The model under review builds one solid part; all positions refer to its coordinate system, in mm. A direction names the side the tool comes from. Round coordinates to 2 decimals unless told otherwise and drop trailing zeros. Write each loop counter-clockwise with the first axis right and the second up, starting at its lowest first coordinate (ties: lowest second). Pieces come first, ordered by that corner, then holes. Notation, with made-up numbers: (17.25, -27) -> (62.25, -27) arc R27 ccw to (62.25, -4) -> close; hole circle Ø4 at (81.5, 64). An arc over 180 degrees is marked (long way). Return JSON: item names as keys, results as strings. Group by question number.
1. Tool access review of faces 1 (the flat face through (11, -3, -15)), 2 (the flat face through (71, -2, 12)): name each direction out of +Z, -Z, +X, -X, +Y, -Y from which nothing blocks a thin tool from reaching the whole face with its end or side.
2. Clearance check with flat-ended pins moving along their axes: P1, Ø3, axis at y = 7.5, z = 6.5, coming from the +X side; P2, Ø6, axis at x = 43, z = 10, coming from the +Y side; P3, Ø16, axis at x = 72, z = 0, coming from the +Y side. State where each tip first meets the part, or that it passes through.
3. Mouldability with a two-part tool opening along Y and no side actions: class faces 3 (the flat face through (11, -3, 15)), 4 (the flat face through (4, -16, 0)), 5 (the cylindrical face through (3, -7, -1)), 6 (the cylindrical face through (12.35, 0.33, -0.21)) as pulls with the +Y half, pulls with the -Y half, needs draft (parallel to the pull), parting line crosses it, or undercut.
4. Take a section at B-B, the plane y = 5. Give the number of separate pieces and of enclosed holes in the cut face, then the cut area to 3 significant figures.
5. Take a section at A-A, the plane x = 71. Write out the cut boundary in (y, z), then the cut area to 3 significant figures.
6. Take a section at C-C, the plane x = -50. Write out the cut boundary in (y, z).
7. For line 1 along Z through (x, y) = (17, -7); line 2 along Z through (x, y) = (75, 6.5); line 3 along X through (y, z) = (-0.5, -11.5), list the stretches that pass through material, from the lowest coordinate up. Write a range as from..to.
from build123d import *

# Parameters (mm, degrees)
CYLINDER006_R               = 2.5
CYLINDER006_DEPTH           = 35
BOX004_W                    = 20
BOX004_H                    = 52
BOX004_DEPTH                = 24
CYLINDER005_R               = 5
CYLINDER005_DEPTH           = 20
CYLINDER005_PLACEMENT_ANGLE = 46
CHAMFER001_SIZE             = 4
CYLINDER004_R               = 2.5
CYLINDER004_DEPTH           = 100
CYLINDER004_PLACEMENT_ANGLE = 46
CYLINDER002_R               = 2
CYLINDER002_DEPTH           = 100
BOX_W                       = 10
BOX_H                       = 40
BOX_DEPTH                   = 100
CYLINDER001_R               = 13
CYLINDER001_DEPTH           = 56
CYLINDER_R                  = 230
CYLINDER_DEPTH              = 100
FUSION_PLACEMENT_ANGLE      = 52.3
FUSION001_PLACEMENT_ANGLE   = 22.4
BOX001_W                    = 49
BOX001_H                    = 54
BOX001_DEPTH                = 100
CYLINDER003_R               = 5
CYLINDER003_DEPTH           = 300
TORUS_R                     = 5
BOX003_W                    = 39
BOX003_H                    = 50
BOX003_DEPTH                = 42
BOX002_W                    = 209
BOX002_H                    = 50
BOX002_DEPTH                = 30
CHAMFER_SIZE                = 15
FILLET_R                    = 2
CHAMFER002_SIZE             = 0.5
CHAMFER003_SIZE             = 1
CHAMFER004_SIZE             = 0.5
CHAMFER005_SIZE             = 1
CHAMFER006_SIZE             = 0.5


with BuildPart() as cylinder006:
    # Cylinder006 → Cylinder006 (new body)
    with BuildSketch(Plane(origin=(10, 0, 3), x_dir=(1, 0, 0), z_dir=(0, -1, 0))):
        Circle(CYLINDER006_R)
    extrude(amount=CYLINDER006_DEPTH)


with BuildPart() as fusion005:
    # Box004 → Box004 (new body)
    with BuildSketch(Plane(origin=(0, -13, -12), x_dir=(1, 0, 0), z_dir=(0, 0, 1))):
        with Locations((10, 26)):
            Rectangle(BOX004_W, BOX004_H)
    extrude(amount=BOX004_DEPTH)

    # Fusion005: union Cylinder006
    add(cylinder006.part)


with BuildPart() as fusion005_1:
    # Fusion005 placement: moved
    add(fusion005.part.moved(Location((61, 0, 0))))


with BuildPart() as chamfer001:
    # Cylinder005 → Cylinder005 (new body)
    with BuildSketch(Plane.XY):
        Circle(CYLINDER005_R)
    extrude(amount=CYLINDER005_DEPTH)


with BuildPart() as chamfer001_1:
    # Cylinder005 placement: moved
    add(chamfer001.part.moved(Location((-52, -8, -20))).rotate(Axis((-52, -8, -20), (0, -1, 0)), CYLINDER005_PLACEMENT_ANGLE))

    # Chamfer001
    chamfer001_edges = [chamfer001_1.edges().sort_by_distance(p)[0] for p in [
        (-69.860088, -8, -9.703532),
    ]]
    chamfer(chamfer001_edges, length=CHAMFER001_SIZE)


with BuildPart() as chamfer001_2:
    # Chamfer001 placement: moved
    add(chamfer001_1.part.moved(Location((-14, 0, 0))))


with BuildPart() as cylinder004:
    # Cylinder004 → Cylinder004 (new body)
    with BuildSketch(Plane.XY):
        Circle(CYLINDER004_R)
    extrude(amount=CYLINDER004_DEPTH)


with BuildPart() as cylinder004_1:
    # Cylinder004 placement: moved
    add(cylinder004.part.moved(Location((-66, -8, -20))).rotate(Axis((-66, -8, -20), (0, -1, 0)), CYLINDER004_PLACEMENT_ANGLE))


with BuildPart() as cylinder002:
    # Cylinder002 → Cylinder002 (new body)
    with BuildSketch(Plane(origin=(106, 11, -34), x_dir=(1, 0, 0), z_dir=(0, 0, 1))):
        Circle(CYLINDER002_R)
    extrude(amount=CYLINDER002_DEPTH)


with BuildPart() as obj1:
    # Box → Box (new body)
    with BuildSketch(Plane(origin=(1000, -30, -50), x_dir=(1, 0, 0), z_dir=(0, 0, 1))):
        with Locations((5, 20)):
            Rectangle(BOX_W, BOX_H)
    extrude(amount=BOX_DEPTH)


with BuildPart() as cylinder001:
    # Cylinder001 → Cylinder001 (new body)
    with BuildSketch(Plane.XZ.offset(-6)):
        Circle(CYLINDER001_R)
    extrude(amount=CYLINDER001_DEPTH)


with BuildPart() as fusion001:
    # Cylinder → Cylinder (new body)
    with BuildSketch(Plane(origin=(0, 230, -50), x_dir=(1, 0, 0), z_dir=(0, 0, 1))):
        Circle(CYLINDER_R)
    extrude(amount=CYLINDER_DEPTH)

    # Fusion: union Cylinder001
    add(cylinder001.part)


with BuildPart() as fusion001_1:
    # Fusion placement: moved
    add(fusion001.part.moved(Location((181.981413, 89.348781, 0))).rotate(Axis((181.981413, 89.348781, 0), (0, 0, 1)), FUSION_PLACEMENT_ANGLE))

    # Fusion001: union obj1
    add(obj1.part)


with BuildPart() as fusion001_2:
    # Fusion001 placement: moved
    add(fusion001_1.part.moved(Location((-87.646187, 17.354412, 0))).rotate(Axis((-87.646187, 17.354412, 0), (0, 0, -1)), FUSION001_PLACEMENT_ANGLE))


with BuildPart() as fusion002:
    # Box001 → Box001 (new body)
    with BuildSketch(Plane(origin=(-141, -28, -50), x_dir=(1, 0, 0), z_dir=(0, 0, 1))):
        with Locations((24.5, 27)):
            Rectangle(BOX001_W, BOX001_H)
    extrude(amount=BOX001_DEPTH)

    # Fusion002: union Fusion001
    add(fusion001_2.part)


with BuildPart() as cylinder003:
    # Cylinder003 → Cylinder003 (new body)
    with BuildSketch(Plane(origin=(-53, -7, 0), x_dir=(0, 0, -1), z_dir=(1, 0, 0))):
        Circle(CYLINDER003_R)
    extrude(amount=CYLINDER003_DEPTH)


with BuildPart() as torus:
    # Torus → Torus (revolve)
    with BuildSketch(Plane(origin=(-53, -7, 30), x_dir=(1, 0, 0), z_dir=(0, 0, -1))):
        with Locations((30, 0)):
            Circle(TORUS_R)
    revolve(axis=Axis((-53, -7, 30), (0, -1, 0)))


with BuildPart() as holes:
    # Box003 → Box003 (new body)
    with BuildSketch(Plane(origin=(-92, -16, -15), x_dir=(1, 0, 0), z_dir=(0, 0, 1))):
        with Locations((19.5, 25)):
            Rectangle(BOX003_W, BOX003_H)
    extrude(amount=BOX003_DEPTH)

    # Common: intersect Torus
    add(torus.part, mode=Mode.INTERSECT)

    # Fusion006: union Cylinder003
    add(cylinder003.part)


with BuildPart() as holes_1:
    # Fusion006 placement: moved
    add(holes.part.moved(Location((0, 0, -6))))

    # Fusion007: union Fusion005, Chamfer001, Cylinder004, Cylinder002, Fusion002
    add(fusion005_1.part)
    add(chamfer001_2.part)
    add(cylinder004_1.part)
    add(cylinder002.part)
    add(fusion002.part)


with BuildPart() as chamfer006:
    # Box002 → Box002 (new body)
    with BuildSketch(Plane(origin=(-92, -16, -15), x_dir=(1, 0, 0), z_dir=(0, 0, 1))):
        with Locations((104.5, 25)):
            Rectangle(BOX002_W, BOX002_H)
    extrude(amount=BOX002_DEPTH)

    # Chamfer
    chamfer_edges = [chamfer006.edges().sort_by_distance(p)[0] for p in [
        (117, -16, 0),
    ]]
    chamfer(chamfer_edges, length=CHAMFER_SIZE)

    # Cut: cut holes
    add(holes_1.part, mode=Mode.SUBTRACT)

    # Fillet
    fillet_edges = [chamfer006.edges().sort_by_distance(p)[0] for p in [
        (117, 31.982324, 13.856394),
        (117, 31.982324, -13.856394),
        (-92, 19.201518, 0),
    ]]
    fillet(fillet_edges, radius=FILLET_R)

    # Chamfer002
    chamfer002_edges = [chamfer006.edges().sort_by_distance(p)[0] for p in [
        (68.5, -16, 3),
        (68.5, -13, 3),
    ]]
    chamfer(chamfer002_edges, length=CHAMFER002_SIZE)

    # Chamfer003
    chamfer003_edges = [chamfer006.edges().sort_by_distance(p)[0] for p in [
        (-86.823069, -7, 15),
        (110.998637, -7.001363, -1),
    ]]
    chamfer(chamfer003_edges, length=CHAMFER003_SIZE)

    # Chamfer004
    chamfer004_edges = [chamfer006.edges().sort_by_distance(p)[0] for p in [
        (104, 11, 15),
        (104, 11, -15),
    ]]
    chamfer(chamfer004_edges, length=CHAMFER004_SIZE)

    # Chamfer005
    chamfer005_edges = [chamfer006.edges().sort_by_distance(p)[0] for p in [
        (-78.375432, -8.003753, -15),
    ]]
    chamfer(chamfer005_edges, length=CHAMFER005_SIZE)

    # Chamfer006
    chamfer006_edges = [chamfer006.edges().sort_by_distance(p)[0] for p in [
        (-92, -7.998647, 1.6325),
    ]]
    chamfer(chamfer006_edges, length=CHAMFER006_SIZE)


solid = chamfer006.part
Output:
{
 "1": {"face 1": "-Z, +X, -X, +Y, -Y", "face 2": "+Y"},
 "2": {"P1": "stops at x = 116.38", "P2": "stops at y = 4.65", "P3": "stops at y = -13"},
 "3": {"face 3": "needs draft", "face 4": "pulls with the -Y half", "face 5": "undercut", "face 6": "pulls with the +Y half"},
 "4": {"separate pieces": "2", "enclosed holes": "1", "area": "2,900 mm^2"},
 "5": {"outline": "(-16, -15) -> (11.23, -15) -> (11.23, -12) -> (-13, -12) -> (-13, 0) -> (-13.5, 0.5) -> (-15.5, 0.5) -> (-16, 0) -> close; (-16, 6) -> (-15.5, 5.5) -> (-13.5, 5.5) -> (-13, 6) -> (-13, 12) -> (11.23, 12) -> (11.23, 15) -> (-16, 15) -> close", "area": "220 mm^2"},
 "6": {"outline": "(-16, -15) -> (5.5, -15) -> (5.5, 15) -> (-16, 15) -> close; hole circle Ø10 at (-7, -6)"},
 "7": {"line 1": "z = -15..-11, -1..15", "line 2": "z = -15..-12, 12..15", "line 3": "x = -92..61, 81..117"}
}
